Could you check a few things on this model? Use its own coordinates, in mm. Face numbers are marked on the shaded views. Give positions to 0.01 mm unless a question says otherwise; leave off trailing zeros. Loops run counter-clockwise (first coordinate to the right, second up) from the corner with the lowest first, then second, coordinate; pieces in that order, holes last. Notation, with made-up numbers: M 71.25,8 L 100.25,8 A34 ccw 100.25,47 Z; hole C 78.25,59 d11. An arc over 180 degrees is marked long. Answer in a Markdown table with one row per item. Add a question column.
1. If we section it at B-B on z = -17: List the corners of the cut face in (x, y) for me, then the cut area to 3 significant figures.
2. I'm going to push flat-ended pins straight in: pin 1 Ø2 at (y, z) = (-9.5, 48.5) entering from -X; pin 2 Ø1.2 at (y, z) = (-5.5, -48.5) entering from +X; pin 3 Ø1.5 at (y, z) = (-9, 20.5) entering from +X. Where does each tip first touch, or does it pass through?
3. Thinking about a two-plate mould opening in Z: for the marked faces 1, 2 and 3, which applies, released by +Z, released by -Z, zero draft, split by the parting line, or undercut?
4. If we section it at A-A on x = -50.5: List the corners of the cut face in (y, z) for me, then the cut area to 3 significant figures.
5. I need wall thicknesses on line 1 along Z through (x, y) = (-23, -9.5); line 2 along X through (y, z) = (-5.5, 37); line 3 along Y through (x, z) = (45, 2.5). Which ranges of each line are inside material? Lowest first, please. Write a range as from..to.
6. If we section it at C-C on y = -7.5: Count the separate pieces of the cut face and the enclosed holes in it, then the cut area to 3 significant figures.
```python
from build123d import *

# Parameters (mm, degrees)
BOSS_EXTRUDE1_DEPTH = 12
SKETCH6_OUTSIDE_W   = 199.812
SKETCH6_OUTSIDE_H   = 139.812
SKETCH6_OUTSIDE_W_2 = 140
SKETCH6_OUTSIDE_H_2 = 2.5
CUT_EXTRUDE1_DEPTH  = 10
SKETCH7_W           = 140
SKETCH7_H           = 80
CUT_EXTRUDE2_DEPTH  = 10
SKETCH13_W          = 6.5
SKETCH13_H          = 10
CUT_EXTRUDE3_DEPTH  = 5
BOSS_EXTRUDE2_DEPTH = 3


with BuildPart() as part:
    # Sketch3 → Boss-Extrude1 (new body)
    with BuildSketch(Plane(origin=(0, 0, 0), x_dir=(1, 0, 0), z_dir=(0, 1, 0))):
        with BuildLine():
            Line((75, -50), (-75, -50))
            ThreePointArc((-75, -50), (-78.535533906, -48.535533906), (-80, -45))
            Line((-80, -45), (-80, 45))
            ThreePointArc((-80, 45), (-78.535533906, 48.535533906), (-75, 50))
            Line((-75, 50), (75, 50))
            ThreePointArc((75, 50), (78.535533906, 48.535533906), (80, 45))
            Line((80, 45), (80, -45))
            ThreePointArc((80, -45), (78.535533906, -48.535533906), (75, -50))
        make_face()
    extrude(amount=-BOSS_EXTRUDE1_DEPTH)

    # Sketch6 outside → Cut-Extrude1 (cut)
    with BuildSketch(Plane.XZ.offset(12)):
        Rectangle(SKETCH6_OUTSIDE_W, SKETCH6_OUTSIDE_H)
        with BuildLine():
            Line((70, -45), (-70, -45))
            ThreePointArc((-70, -45), (-73.535533906, -43.535533906), (-75, -40))
            Line((-75, -40), (-75, 40))
            ThreePointArc((-75, 40), (-73.535533906, 43.535533906), (-70, 45))
            Line((-70, 45), (70, 45))
            ThreePointArc((70, 45), (73.535533906, 43.535533906), (75, 40))
            Line((75, 40), (75, -40))
            ThreePointArc((75, -40), (73.535533906, -43.535533906), (70, -45))
        make_face(mode=Mode.SUBTRACT)
        with Locations((0, 48.75)):
            Rectangle(SKETCH6_OUTSIDE_W_2, SKETCH6_OUTSIDE_H_2, mode=Mode.SUBTRACT)
        with Locations((0, -48.75)):
            Rectangle(SKETCH6_OUTSIDE_W_2, SKETCH6_OUTSIDE_H_2, mode=Mode.SUBTRACT)
    extrude(amount=-CUT_EXTRUDE1_DEPTH, mode=Mode.SUBTRACT)

    # Sketch7 → Cut-Extrude2 (cut)
    with BuildSketch(Plane.XZ.offset(12)):
        Rectangle(SKETCH7_W, SKETCH7_H)
    extrude(amount=-CUT_EXTRUDE2_DEPTH, mode=Mode.SUBTRACT)

    # Sketch13 → Cut-Extrude3 (cut)
    with BuildSketch(Plane(origin=(0, 0, -50), x_dir=(-1, 0, 0), z_dir=(0, 0, -1))):
        with Locations((0, -7)):
            Rectangle(SKETCH13_W, SKETCH13_H)
    cut_extrude3 = extrude(amount=-CUT_EXTRUDE3_DEPTH, mode=Mode.SUBTRACT)

    # Sketch14 → Boss-Extrude2 (add, symmetric)
    with BuildSketch(Plane(origin=(0, 0, 0), x_dir=(0, 0, -1), z_dir=(1, 0, 0))):
        Polygon((50, -2), (50, -5.8), (50, -10), (49.25, -10), (49.25, -5.85), (48.5, -5.1), (48.5, -4.6), (49, -4.6), (49, -2), align=None)
    boss_extrude2 = extrude(amount=BOSS_EXTRUDE2_DEPTH, both=True)

    # Mirror1: Cut-Extrude3, Boss-Extrude2 across plane
    add(cut_extrude3.mirror(Plane.XY), mode=Mode.SUBTRACT)
    add(boss_extrude2.mirror(Plane.XY))


solid = part.part
```
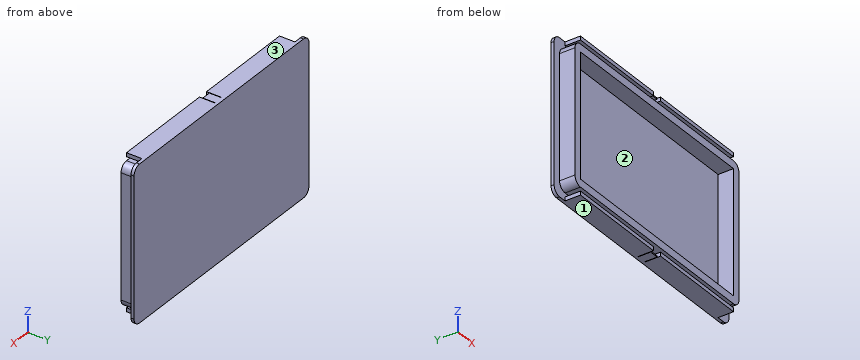
Results:
| question | item | result |
|---|---|---|
| 1 | outline | M -80,-2 L -75,-2 L -75,-12 L -70,-12 L -70,-2 L 70,-2 L 70,-12 L 75,-12 L 75,-2 L 80,-2 L 80,0 L -80,0 Z |
| 1 | area | 420 mm2 |
| 2 | pin 1 | x = -70 |
| 2 | pin 2 | x = 70 |
| 2 | pin 3 | x = 75 |
| 3 | face 1 | released by -Z |
| 3 | face 2 | undercut |
| 3 | face 3 | released by +Z |
| 4 | outline | M -12,-50 L 0,-50 L 0,50 L -12,50 L -12,47.5 L -2,47.5 L -2,45 L -12,45 L -12,40 L -2,40 L -2,-40 L -12,-40 L -12,-45 L -2,-45 L -2,-47.5 L -12,-47.5 Z |
| 4 | area | 350 mm2 |
| 5 | line 1 | -50..-47.5, -45..-40, 40..45, 47.5..50 |
| 5 | line 2 | -75..-70, 70..75 |
| 5 | line 3 | -2..0 |
| 6 | separate pieces | 7 |
| 6 | enclosed holes | 1 |
| 6 | area | 2,960 mm2 |
